Work out the finished part from the listing and answer in its coordinate system (mm). A direction names the side the tool comes from. Round coordinates to 2 decimals unless told otherwise and drop trailing zeros. Order: outer loops, then holes, each group sorted by start corner. A loop starts at its lowest first (then second) coordinate and runs counter-clockwise, first axis right, second up. Notation, with made-up numbers: M -4.75,-16 L 54.25,-16 A16 ccw 54.25,6 Z; hole C -3.5,44.25 d5. An arc over 180 degrees is marked long. Return JSON: item names as keys, results as strings.
from build123d import *

# Parameters (mm, degrees)
F4_D     = 3.3
F4_DEPTH = 8.1
F4_START = 0.0779595
F4_TIP   = 0.9914200214
F5_SIZE  = 0.75


with BuildPart() as f1:
    # F0 (on Front) → F1 (revolve)
    with BuildSketch(Plane.XZ):
        Polygon((0, 14.325), (0, 17.5), (-60, 17.5), (-60, 14.325), (-140, 14.325), (-140, 12), (-56, 12), (-56, 14.325), align=None)
    revolve(axis=Axis((-73.5066011898, 0, 0), (-1, 0, 0)))

    # F4
    # its depths count from where the whole tool has entered the part; down to there all is cleared
    with Locations(Plane.XY.offset(17.5).offset(-F4_START)):
        with Locations((-25, 0)):
            Hole(F4_D / 2, depth=F4_DEPTH)
            with Locations((0, 0, -(F4_DEPTH + F4_TIP / 2))):  # 118° drill point
                Cone(0, F4_D / 2, F4_TIP, mode=Mode.SUBTRACT)

    # F5
    f5_edges = [f1.edges().sort_by_distance(p)[0] for p in [
        (-140, 0, -14.325),
        (-140, 0, -12),
        (-60, 0, -17.5),
        (0, 0, -17.5),
        (0, 0, -14.325),
        (-56, 0, -12),
    ]]
    chamfer(f5_edges, length=F5_SIZE)


solid = f1.part
Item 1: Which of the six approach directions +Z, -Z, +X, -X, +Y, -Y give full straight-line access (tool end or side, diameter ignored) to faces 1 (the flat face through (-60, 5, 14)), 2 (the cylindrical face through (-23.35, 0.07, 15.84)), 3 (the cylindrical face through (-27.988, 4.303, 13.663))?
Output:
{"face 1": "-X", "face 2": "+Z", "face 3": "+X"}
Item 2: Consider line 1 along Y through (x, z) = (-19.5, 0) (3 decimals); line 2 along X through (y, z) = (0, 15.5); line 3 along Z through (x, y) = (-27, 3). Determine where each line is inside the solid, lowest interval first. Write a range as [from, to].
Output:
{"line 1": "y = [-17.5, -14.325], [14.325, 17.5]", "line 2": "x = [-60, -26.65], [-23.35, 0]", "line 3": "z = [-17.24, -14.01], [14.01, 17.24]"}
Item 3: Find section C-C (x = -21.5). Determine the outline of the cut face in (y, z) (3 decimals), plus the area to 3 significant figures.
Output:
{"outline": "C 0,0 d35; hole C 0,0 d28.65", "area": "317 mm^2"}
Item 4: Find section A-A (y = 0). State how many separate pieces and enclosed holes the cut face has, plus the area to 3 significant figures.
Output:
{"separate pieces": "3", "enclosed holes": "0", "area": "758 mm^2"}
Item 5: Find section B-B (z = 0). Determine the outline of the cut face in (x, y) (3 decimals), plus the area to 3 significant figures.
Output:
{"outline": "M -140,-13.575 L -139.25,-14.325 L -60,-14.325 L -60,-16.75 L -59.25,-17.5 L -0.75,-17.5 L 0,-16.75 L 0,-15.075 L -0.75,-14.325 L -56,-14.325 L -56,-12.75 L -56.75,-12 L -139.25,-12 L -140,-12.75 Z; M -140,12.75 L -139.25,12 L -56.75,12 L -56,12.75 L -56,14.325 L -0.75,14.325 L 0,15.075 L 0,16.75 L -0.75,17.5 L -59.25,17.5 L -60,16.75 L -60,14.325 L -139.25,14.325 L -140,13.575 Z", "area": "768 mm^2"}
Item 6: Find section D-D (x = -125). Determine the outline of the cut face in (y, z) (3 decimals).
Output:
{"outline": "C 0,0 d28.65; hole C 0,0 d24"}
Item 7: Each of these flat-tipped pins is pushed along its axis until it touches: pin 1 (14.5 mm diameter, centred on y = 1.5, z = 2, fed in from +X); pin 2 (8 mm diameter, centred on y = 6.5, z = -12, fed in from -X); pin 3 (1.5 mm diameter, centred on x = -47, z = -8, fed in from +Y); pin 4 (10 mm diameter, centred on x = -92.5, z = 4.5, fed in from -Y) (3 decimals). Where does it stop, or does it pass through?
Output:
{"pin 1": "passes through", "pin 2": "stops at x = -140", "pin 3": "stops at y = 15.93", "pin 4": "stops at y = -14.325"}
Item 8: The mould has two halves that part along Z. Classify faces 4 (the cylindrical face through (-100.18, 4.303, 13.663)), 5 (the flat face through (-56, -1, 13)), 6 (the flat face through (0, 6, 14)): pulls with the +Z half, pulls with the -Z half, needs draft (parallel to the pull), parting line crosses it, or undercut.
Output:
{"face 4": "parting line crosses it", "face 5": "undercut", "face 6": "needs draft"}
